Source: CAD feature listing. Evaluate the final solid. Frame: model axes, mm. A direction names the side the tool comes from. Give positions to 0.01 mm unless a question says otherwise; leave off trailing zeros. Order: outer loops, then holes, each group sorted by start corner. A loop starts at its lowest first (then second) coordinate and runs counter-clockwise, first axis right, second up.
from build123d import *

# Parameters (mm, degrees)
EXTRUDE_1_DEPTH = 19
SKETCH_2_R      = 4.5
EXTRUDE_2_DEPTH = 12.2
EXTRUDE_3_DEPTH = 15


with BuildPart() as part:
    # 草图1 → 拉伸1 (new body)
    with BuildSketch(Plane(origin=(0, 0, 0), x_dir=(0, 0, -1), z_dir=(1, 0, 0))):
        with BuildLine():
            Line((-2.179449472, 4.5), (2.179449472, 4.5))
            ThreePointArc((2.179449472, 4.5), (0, -5), (-2.179449472, 4.5))
        make_face()
    extrude(amount=EXTRUDE_1_DEPTH)

    # 草图2 → 拉伸2 (add)
    with BuildSketch(Plane(origin=(19, 0, 0), x_dir=(0, 0, -1), z_dir=(1, 0, 0))):
        with Locations(Location((0, 0, 0), (0, 0, 90))):
            Circle(SKETCH_2_R)
    extrude(amount=EXTRUDE_2_DEPTH)

    # 草图3 → 拉伸3 (add)
    with BuildSketch(Plane(origin=(31.2, 0, 0), x_dir=(0, 0, -1), z_dir=(1, 0, 0))):
        with BuildLine():
            Line((-1.936491673, 3.5), (1.936491673, 3.5))
            ThreePointArc((1.936491673, 3.5), (0, -4), (-1.936491673, 3.5))
        make_face()
    extrude(amount=EXTRUDE_3_DEPTH)


solid = part.part
1) Section query A-A on y = 0. Output: boundary loops of the cut face in (x, z), and give its area (3 significant figures).
Checks:
outline: (0, -5) - (19, -5) - (19, -4.5) - (31.2, -4.5) - (31.2, -4) - (46.2, -4) - (46.2, 4) - (31.2, 4) - (31.2, 4.5) - (19, 4.5) - (19, 5) - (0, 5) - close
area: 420 mm2
2) Reachability of faces 1 (the face through (25.015, 4.292, 1.352)), 2 (the face through (46.2, 0, 0)), 3 (the face through (39, 3.5, 0)) from +Z, -Z, +X, -X, +Y, -Y: full face, straight path, thin tool, end or side. Return the list, or none.
Checks:
face 1: +X
face 2: +Z, -Z, +X, +Y, -Y
face 3: +Z, -Z, +X, +Y
3) Section query B-B on z = -0.75. Output: boundary loops of the cut face in (x, y), and give its area (3 significant figures).
Checks:
outline: (0, -4.94) - (19, -4.94) - (19, -4.44) - (31.2, -4.44) - (31.2, -3.93) - (46.2, -3.93) - (46.2, 3.5) - (31.2, 3.5) - (31.2, 4.44) - (19, 4.44) - (19, 4.5) - (0, 4.5) - close
area: 399 mm2
4) Section query C-C on x = 13.5. Output: boundary loops of the cut face in (y, z).
Checks:
outline: (4.5, -2.18) - (4.5, 2.18) arc R5 ccw (long way) to start
5) First-contact query: pin 1 Ø1.2 at (x, z) = (42.5, -0.5) entering from +Y; pin 2 Ø4 at (x, z) = (30, 0.5) entering from -Y. Flat tips, straight axial feed; report the tip coordinate or a pass-through.
Checks:
pin 1: stops at y = 3.5
pin 2: stops at y = -4.5
6) Section query D-D on x = 39. Output: boundary loops of the cut face in (y, z).
Checks:
outline: (3.5, -1.94) - (3.5, 1.94) arc R4 ccw (long way) to start
7) Ray query, L1, parallel to Z at x = 43, y = -3.5; L2, parallel to X at y = 3, z = -3; L3, parallel to Z at x = 18.5, y = -0.25. Return the intervals inside material, ascending.
Checks:
L1: z = -1.94 to 1.94
L2: x = 0 to 31.2
L3: z = -4.99 to 4.99
